Input: part model. Units: mm. Frame: model coordinates. A direction names the side the tool comes from. Give positions to 0.01 mm unless a question says otherwise; leave off trailing zeros. Write each loop counter-clockwise with the first axis right and the second up, starting at its lowest first coordinate (ties: lowest second). Pieces come first, ordered by that corner, then holes. Notation, with made-up numbers: (-25.75, 32) -> (29.25, 32) arc R14 ccw to (29.25, 40) -> close; hole circle Ø10 at (60, 60). An arc over 180 degrees is marked (long way). Return JSON: item names as keys, results as strings. Group by question number.
Item 1: Mould query, pull axis X, two halves, no side actions, for faces 1 (the face through (156.911, 30, 5)), 2 (the face through (-95.94, 56.99, 4.93)), 3 (the face through (132, 60, 5)). Classes: released by +X, released by -X, zero draft, split by the parting line, or undercut.
Item 2: Section A-A, the plane z = 7. Count the separate pieces of the cut face and the enclosed holes in it, then the cut area to 3 significant figures.
Item 3: Line query: line 1 (X direction, y = 46.5, z = 3.5); line 2 (Y direction, x = 76, z = 8.25); line 3 (Y direction, x = -102.5, z = 3.5). Output: solid intervals per line, ascending. Write a range as [from, to].
Item 4: Pin query (flat end, axial travel): P1, Ø1, axis at x = 25.5, z = 9, coming from the +Y side. Return the tip coordinate at first contact, or that it passes through.
Item 5: Section B-B, the plane x = -18.5. Return loops of the section in (y, z).
Item 6: Set-up query: faces 4 (the face through (6, 6, 5)), 5 (the face through (-118, 60, 5)), 6 (the face through (109.92, 57.15, 4.93)). Return all of +Z, -Z, +X, -X, +Y, -Y with unobstructed straight access to the full face (end or side cutting, diameter ignored); none if empty.
from build123d import *

# Parameters (mm, degrees)
MODEL_R             = 4.05
MODEL_R_2           = 3
MODEL_R_3           = 2
BOSS_EXTRUDE1_DEPTH = 10


with BuildPart() as part:
    # Model → Boss-Extrude1 (new body)
    with BuildSketch(Plane.XY):
        with BuildLine():
            Line((-90.089430894, 6), (103.910569106, 6))
            ThreePointArc((103.910569106, 6), (106.031889449, 5.121320344), (106.910569106, 3))
            ThreePointArc((106.910569106, 3), (107.789248762, 0.878679656), (109.910569106, 0))
            Line((109.910569106, 0), (146.910569106, 0))
            ThreePointArc((146.910569106, 0), (153.981636918, 2.928932188), (156.910569106, 10))
            Line((156.910569106, 10), (156.910569106, 50))
            ThreePointArc((156.910569106, 50), (153.981636918, 57.071067812), (146.910569106, 60))
            Line((146.910569106, 60), (116.910569106, 60))
            ThreePointArc((116.910569106, 60), (109.839501294, 57.071067812), (106.910569106, 50))
            Line((106.910569106, 50), (106.910569106, 40))
            ThreePointArc((106.910569106, 40), (103.981636918, 32.928932188), (96.910569106, 30))
            Line((96.910569106, 30), (-83.089430894, 30))
            ThreePointArc((-83.089430894, 30), (-90.160498706, 32.928932188), (-93.089430894, 40))
            Line((-93.089430894, 40), (-93.089430894, 50))
            ThreePointArc((-93.089430894, 50), (-96.018363082, 57.071067812), (-103.089430894, 60))
            Line((-103.089430894, 60), (-133.089430894, 60))
            ThreePointArc((-133.089430894, 60), (-140.160498706, 57.071067812), (-143.089430894, 50))
            Line((-143.089430894, 50), (-143.089430894, 10))
            ThreePointArc((-143.089430894, 10), (-140.160498706, 2.928932188), (-133.089430894, 0))
            Line((-133.089430894, 0), (-96.089430894, 0))
            ThreePointArc((-96.089430894, 0), (-93.968110551, 0.878679656), (-93.089430894, 3))
            ThreePointArc((-93.089430894, 3), (-92.210751238, 5.121320344), (-90.089430894, 6))
        make_face()
        with Locations((131.910569106, 30)):
            Circle(MODEL_R, mode=Mode.SUBTRACT)
        with Locations((-118.089430894, 30)):
            Circle(MODEL_R_2, mode=Mode.SUBTRACT)
        with Locations((6.910569106, 18)):
            Circle(MODEL_R_3, mode=Mode.SUBTRACT)
        with Locations((-33.089430894, 18)):
            Circle(MODEL_R_3, mode=Mode.SUBTRACT)
        with Locations((-13.089430894, 18)):
            Circle(MODEL_R_3, mode=Mode.SUBTRACT)
        with Locations((86.910569106, 18)):
            Circle(MODEL_R_3, mode=Mode.SUBTRACT)
        with Locations((66.910569106, 18)):
            Circle(MODEL_R_3, mode=Mode.SUBTRACT)
        with Locations((46.910569106, 18)):
            Circle(MODEL_R_3, mode=Mode.SUBTRACT)
        with Locations((26.910569106, 18)):
            Circle(MODEL_R_3, mode=Mode.SUBTRACT)
        with Locations((146.910569106, 10)):
            Circle(MODEL_R_3, mode=Mode.SUBTRACT)
        with Locations((146.910569106, 50)):
            Circle(MODEL_R_3, mode=Mode.SUBTRACT)
        with Locations((-133.089430894, 10)):
            Circle(MODEL_R_3, mode=Mode.SUBTRACT)
        with Locations((-133.089430894, 50)):
            Circle(MODEL_R_3, mode=Mode.SUBTRACT)
        with Locations((-93.089430894, 18)):
            Circle(MODEL_R_3, mode=Mode.SUBTRACT)
        with Locations((-73.089430894, 18)):
            Circle(MODEL_R_3, mode=Mode.SUBTRACT)
        with Locations((-53.089430894, 18)):
            Circle(MODEL_R_3, mode=Mode.SUBTRACT)
        with Locations((116.910569106, 50)):
            Circle(MODEL_R_3, mode=Mode.SUBTRACT)
        with Locations((116.910569106, 10)):
            Circle(MODEL_R_3, mode=Mode.SUBTRACT)
    extrude(amount=BOSS_EXTRUDE1_DEPTH)


solid = part.part
Answer below:
{
 "1": {"face 1": "released by +X", "face 2": "undercut", "face 3": "zero draft"},
 "2": {"separate pieces": "1", "enclosed holes": "18", "area": "10,400 mm2"},
 "3": {"line 1": "x = [-143.09, -93.09], [106.91, 156.91]", "line 2": "y = [6, 30]", "line 3": "y = [0, 59.98]"},
 "4": {"P1": "stops at y = 30"},
 "5": {"outline": "(6, 0) -> (30, 0) -> (30, 10) -> (6, 10) -> close"},
 "6": {"face 4": "+Z, -Z, -Y", "face 5": "+Z, -Z, +X, -X, +Y", "face 6": "+Z, -Z, +Y"}
}
